Source: CAD feature listing. Evaluate the final solid. Frame: model axes, mm. A direction names the side the tool comes from. Coordinates: 2 decimals unless noted, no trailing zeros. Loops run counter-clockwise (first coordinate to the right, second up) from the corner with the lowest first, then second, coordinate; pieces in that order, holes last. Notation, with made-up numbers: (20.25, 30) -> (66.25, 30) arc R22 ccw to (66.25, 69) -> close; hole circle Ø4 at (34, 29.25). An arc over 180 degrees is marked (long way). Answer as a JSON object with one key per item and string values. Group by question number.
from build123d import *

# Parameters (mm, degrees)
ESQUISSE1_R             = 20
BOSS_EXTRU_1_DEPTH      = 20
TROU_TARAUD_M61_D       = 5
TROU_TARAUD_M61_DEPTH   = 17
TROU_TARAUD_M61_TIP     = 1.502151548
ENL_V_MAT_EXTRU_1_DEPTH = 25


with BuildPart() as part:
    # Esquisse1 → Boss.-Extru.1 (new body)
    with BuildSketch(Plane.XY):
        Circle(ESQUISSE1_R)
    extrude(amount=BOSS_EXTRU_1_DEPTH)

    # Trou taraudé M61
    with Locations(Plane(origin=(19.999953956, 0.042915747, 10), x_dir=(-0.002145787, 0.999997698, 0), z_dir=(0.999997698, 0.002145787, 0))):
        with Locations((0, 0)):
            Hole(TROU_TARAUD_M61_D / 2, depth=TROU_TARAUD_M61_DEPTH)
            with Locations((0, 0, -(TROU_TARAUD_M61_DEPTH + TROU_TARAUD_M61_TIP / 2))):  # 118° drill point
                Cone(0, TROU_TARAUD_M61_D / 2, TROU_TARAUD_M61_TIP, mode=Mode.SUBTRACT)

    # Esquisse11 → Enlèv. mat.-Extru.1 (cut)
    with BuildSketch(Plane.XY.offset(20)):
        with BuildLine():
            Line((3, 9.539392014), (3, 12.039392014))
            Line((3, 12.039392014), (-3, 12.039392014))
            Line((-3, 12.039392014), (-3, 9.539392014))
            ThreePointArc((-3, 9.539392014), (0, -10), (3, 9.539392014))
        make_face()
    extrude(amount=-ENL_V_MAT_EXTRU_1_DEPTH, mode=Mode.SUBTRACT)


solid = part.part
1. Ray query, L1, parallel to Y at x = 0, z = 14; L2, parallel to Y at x = 9, z = 12.5; L3, parallel to X at y = -7, z = 2 (3 decimals). Return the intervals inside material, ascending.
2. Section query C-C on y = -8. Return loops of the section in (x, z), then the cut area to 3 significant figures.
3. Mould query, pull axis X, two halves, no side actions, for faces 1 (the face through (3, 11, 10)), 2 (the face through (-4.336, -19.524, 9.86)), 3 (the face through (-5, 9, 20)). Classes: pulls with the +X half, pulls with the -X half, needs draft (parallel to the pull), parting line crosses it, or undercut.
4. Section query D-D on x = -10.5. Return loops of the section in (y, z), then the cut area to 3 significant figures.
5. Reachability of faces 4 (the face through (-5, 9, 0)), 5 (the face through (-3, 11, 10)) from +Z, -Z, +X, -X, +Y, -Y: full face, straight path, thin tool, end or side. Return the list, or none.
6. Section query B-B on z = 6. Return loops of the section in (x, y), then the cut area to 3 significant figures.
7. Pin query (flat end, axial travel): pin 1 Ø8 at (x, z) = (-9.5, 3) entering from +Y; pin 2 Ø6 at (x, z) = (-12, 11.5) entering from -Y; pin 3 Ø1.5 at (y, z) = (-10.5, 16.5) entering from +X. Return the tip coordinate at first contact, or that it passes through.
8. Section query A-A on x = 0. Return loops of the section in (y, z), then the cut area to 3 significant figures.
Solved:
{
 "1": {"L1": "-20 to -10, 12.04 to 20", "L2": "-17.86 to -4.36, 4.36 to 17.86", "L3": "-18.735 to -7.141, 7.141 to 18.735"},
 "2": {"outline": "(-18.33, 0) -> (-6, 0) -> (-6, 20) -> (-18.33, 20) -> close; (6, 0) -> (18.33, 0) -> (18.33, 20) -> (6, 20) -> close", "area": "493 mm^2"},
 "3": {"face 1": "undercut", "face 2": "parting line crosses it", "face 3": "needs draft"},
 "4": {"outline": "(-17.02, 0) -> (17.02, 0) -> (17.02, 20) -> (-17.02, 20) -> close", "area": "681 mm^2"},
 "5": {"face 4": "-Z, +X, -X, +Y, -Y", "face 5": "+Z, -Z"},
 "6": {"outline": "circle Ø40 at (0, 0); hole (-3, 9.54) arc R10 ccw (long way) to (3, 9.54) -> (3, 12.04) -> (-3, 12.04) -> close", "area": "929 mm^2"},
 "7": {"pin 1": "y = 19.23", "pin 2": "y = -17.86", "pin 3": "x = 17.46"},
 "8": {"outline": "(-20, 0) -> (-10, 0) -> (-10, 20) -> (-20, 20) -> close; (12.04, 0) -> (20, 0) -> (20, 20) -> (12.04, 20) -> close", "area": "359 mm^2"}
}
